The figure shows three views and two pictorial views of one solid part (mm, origin at its lowest corner). Answer the questions. A direction names the side the tool comes from. Coordinates: 2 decimals unless noted, no trailing zeros. Write each loop counter-clockwise with the first axis right and the second up, starting at its lowest first coordinate (ties: lowest second). Pieces come first, ordered by that corner, then holes.
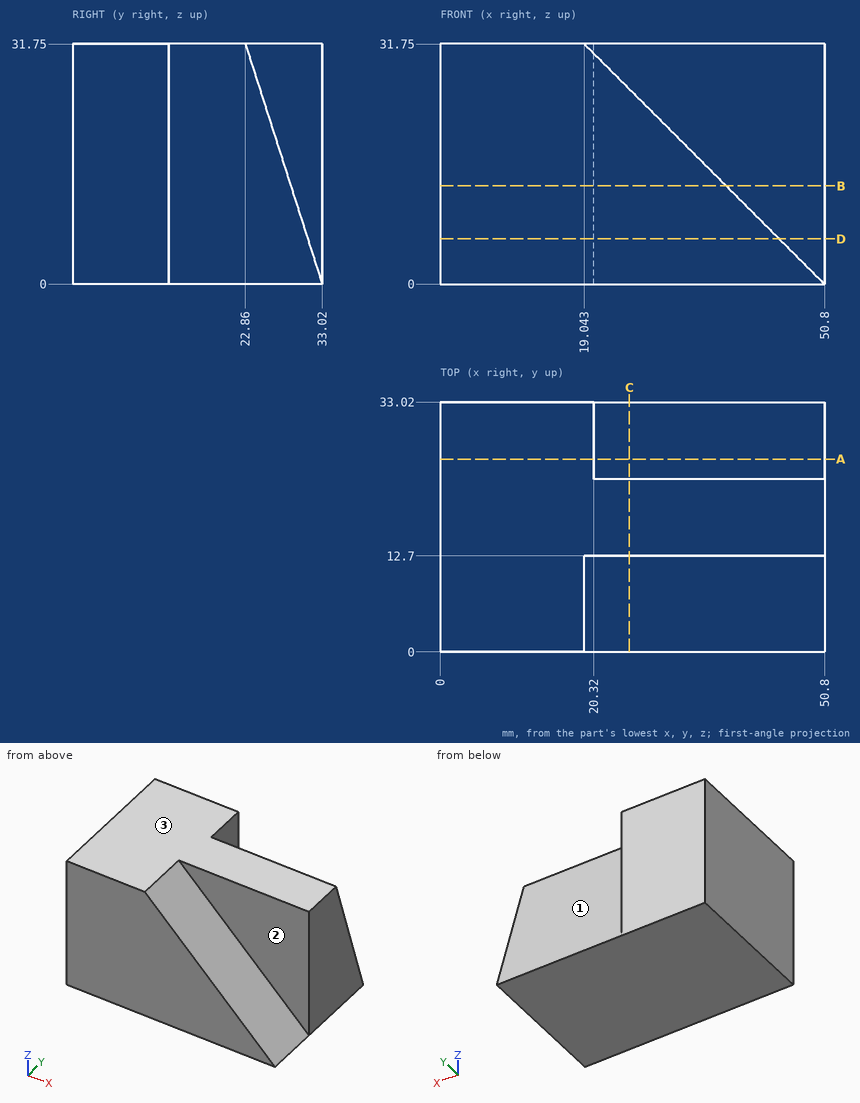
1. Find the intervals of material crossed by L1, parallel to X at y = 31, z = 17.5; L2, parallel to Y at x = 23, z = 22.5; L3, parallel to Z at x = 28, y = 6 (1 decimal), in increasing order.
Results found:
L1: x = 0 to 20.32
L2: y = 0 to 25.82
L3: z = 0 to 22.8
2. Section C-C on x = 25 is taken. Give the vertices of the cut face in (y, z).
Results found:
outline: (0, 0) - (33.02, 0) - (22.86, 31.75) - (12.7, 31.75) - (12.7, 25.79) - (0, 25.79) - close
3. Section D-D on z = 6 is taken. Give the vertices of the cut face in (x, y), then the cut area to 3 significant figures.
Results found:
outline: (0, 0) - (44.8, 0) - (44.8, 12.7) - (50.8, 12.7) - (50.8, 31.1) - (20.32, 31.1) - (20.32, 33.02) - (0, 33.02) - close
area: 1,540 mm2
4. A tool of negligible diameter and unlimited length cuts with its end or side. For the marked faces 1, 2 and 3, from which of +Z, -Z, +X, -X, +Y, -Y can it reach the whole face along a straight path? Write none if from no direction.
Results found:
face 1: +Z, +X, +Y
face 2: +Z, +X, -Y
face 3: +Z, +X, -X, +Y, -Y
5. Section B-B on z = 13 is taken. Give the vertices of the cut face in (x, y), then the cut area to 3 significant figures.
Results found:
outline: (0, 0) - (37.8, 0) - (37.8, 12.7) - (50.8, 12.7) - (50.8, 28.86) - (20.32, 28.86) - (20.32, 33.02) - (0, 33.02) - close
area: 1,390 mm2
6. Flat-ended cylindrical pins translate along their axes: P1, Ø12, axis at x = 38.5, z = 13.5, coming from the +Y side; P2, Ø6, axis at x = 30, z = 5.5, coming from the -Y side. Find the tip coordinate at first contact, or state that the pin passes through.
Results found:
P1: stops at y = 30.62
P2: stops at y = 0
7. Section A-A on y = 25.5 is taken. Give the vertices of the cut face in (x, z), then the cut area to 3 significant figures.
Results found:
outline: (0, 0) - (50.8, 0) - (50.8, 23.5) - (20.32, 23.5) - (20.32, 31.75) - (0, 31.75) - close
area: 1,360 mm2
